The model under review builds one solid part; all positions refer to its coordinate system, in mm. Face numbers are marked on the shaded views. A direction names the side the tool comes from. Coordinates: 2 decimals unless noted, no trailing zeros. Order: outer loops, then holes, each group sorted by start corner. A loop starts at its lowest first (then second) coordinate and runs counter-clockwise, first axis right, second up. Notation, with made-up numbers: (-28, 82) -> (4, 82) arc R21 ccw to (4, 95) -> close; hole circle Ø6 at (60, -12.75). An arc over 180 degrees is marked (long way). Put each result on its own line as item: value.
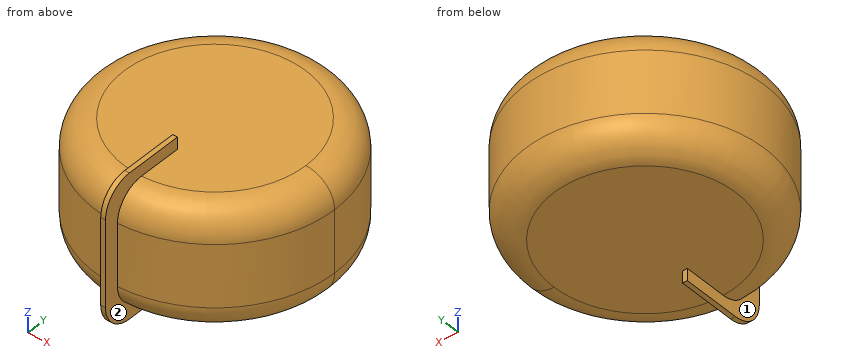
from build123d import *

# Parameters (mm, degrees)
F0_R     = 25
F1_DEPTH = 12.5
F2_R     = 6
F4_DEPTH = 0.5


with BuildPart() as f1:
    # F0 (on Top) → F1 (new body, symmetric)
    with BuildSketch(Plane.XY):
        Circle(F0_R)
    extrude(amount=F1_DEPTH, both=True)

    # F2
    f2_edges = [f1.edges().sort_by_distance(p)[0] for p in [
        (-25, 0, 12.5),
        (-25, 0, -12.5),
    ]]
    fillet(f2_edges, radius=F2_R)

    # F3 (on Right) → F4 (join, symmetric)
    with BuildSketch(Plane.YZ):
        with BuildLine():
            Line((-22, -15), (-10, -15))
            Line((-10, -15), (-10, 15))
            Line((-10, 15), (-22, 15))
            ThreePointArc((-22, 15), (-26.242641, 13.242641), (-28, 9))
            Line((-28, 9), (-28, -9))
            ThreePointArc((-28, -9), (-26.242641, -13.242641), (-22, -15))
        make_face()
    extrude(amount=F4_DEPTH, both=True)


solid = f1.part
Item 1: For pin 1 Ø14.5 at (y, z) = (-22.5, -3.5) entering from +X; pin 2 Ø3 at (x, z) = (-11, -10) entering from +Y; pin 3 Ø2 at (x, z) = (-14.5, 7.5) entering from +Y, all flat-tipped, find the tip position at first contact; note any pin that passes through.
Answers below:
pin 1: x = 19.81
pin 2: y = 22.37
pin 3: y = 20.97
Item 2: For the marked faces 1 and 2, list the 3-axis set-ups (+Z, -Z, +X, -X, +Y, -Y) from which the entire face can be reached by the end or side of a thin tool; tool diameter is ignored.
Answers below:
face 1: -X, -Y
face 2: +X, -Y
Item 3: Consider section A-A on z = 2.5. Write out the cut boundary in (x, y) (3 decimals).
Answers below:
outline: (-0.5, -28) -> (0.5, -28) -> (0.5, -24.995) arc R25 ccw (long way) to (-0.5, -24.995) -> close
Item 4: Consider section B-B on z = 8. Write out the cut boundary in (x, y), and give its area (3 significant figures).
Answers below:
outline: (-0.5, -28) -> (0.5, -28) -> (0.5, -24.8) arc R24.81 ccw (long way) to (-0.5, -24.8) -> close
area: 1,940 mm^2
Item 5: For line 1 (Z direction, x = 7, y = -14); line 2 (X direction, y = 20, z = -6); line 3 (X direction, y = -23.5, z = 12), list the stretches that pass through material, from the lowest coordinate up. Write a range as from..to.
Answers below:
line 1: -12.5..12.5
line 2: -15..15
line 3: -0.5..0.5
